```python
from build123d import *

# Parameters (mm, degrees)
F0_W     = 110
F0_H     = 110
F1_DEPTH = 25
F1_TAPER = -11
F2_R     = 25
F3_DEPTH = 22
F4_W     = 120
F4_H     = 120
F4_R     = 25
F5_DEPTH = 25
F5_TAPER = -11


with BuildPart() as f1:
    # F0 (on Top) → F1 (new body)
    with BuildSketch(Plane.XY):
        with Locations((55, 55)):
            Rectangle(F0_W, F0_H)
    extrude(amount=F1_DEPTH, taper=F1_TAPER)

    # F2 (on face) → F3 (join)
    with BuildSketch(Plane.XY.offset(25)):
        with Locations((55, 55)):
            Circle(F2_R)
    extrude(amount=F3_DEPTH)

    # F4 (on face) → F5 (join)
    with BuildSketch(Plane.XY.offset(47)):
        with Locations((55.1147708297, 55.155566372)):
            Rectangle(F4_W, F4_H)
        with Locations((55, 55)):
            Circle(F4_R, mode=Mode.SUBTRACT)
        with Locations((55, 55)):
            Circle(F4_R)
    extrude(amount=F5_DEPTH, taper=F5_TAPER)


solid = f1.part
```
Part model, mm, in its own coordinate system. Round coordinates to 2 decimals unless told otherwise and drop trailing zeros. Loops run counter-clockwise (first coordinate to the right, second up) from the corner with the lowest first, then second, coordinate; pieces in that order, holes last. Notation, with made-up numbers: (80, 67) -> (95, 67) arc R23 cw to (95, 95) -> close; hole circle Ø6 at (71, -7). An arc over 180 degrees is marked (long way). Use one line per item in the form item = value. Start each with the question number.
Item 1: Drill centre lines: line 1 along Z through (x, y) = (31, 17); line 2 along Y through (x, z) = (66, 67.5); line 3 along Y through (x, z) = (52, 43). Where is each one in solid material? Low to high.
Item 2: Band-saw the part on A-A (z = 27). List the corners of the cut face in (x, y).
Item 3: Two-plate mould, pull along Z, no slides. Class faces 1 (the flat face through (27, 55, 25)), 2 (the flat face through (53, 55, 72)), 3 (the flat face through (53, 55, 0)): released by +Z, released by -Z, zero draft, split by the parting line, or undercut.
Item 4: Drop flat-ended pins along their axis: pin 1 Ø4 at (x, z) = (73, 14.5) entering from +Y; pin 2 Ø5 at (x, z) = (48, 42.5) entering from -Y; pin 3 Ø2 at (y, z) = (13.5, 60.5) entering from +X; pin 4 Ø5 at (y, z) = (96.5, 29) entering from -X. Give the stop position or say it passes through.
Data:
q1.line_1 = 0 to 25, 47 to 72
q1.line_2 = -8.83 to 119.14
q1.line_3 = 30.18 to 79.82
q2.outline = circle Ø50 at (55, 55)
q3.face_1 = undercut
q3.face_2 = released by +Z
q3.face_3 = released by -Z
q4.pin_1 = 113.21
q4.pin_2 = 30.41
q4.pin_3 = 117.93
q4.pin_4 = through
